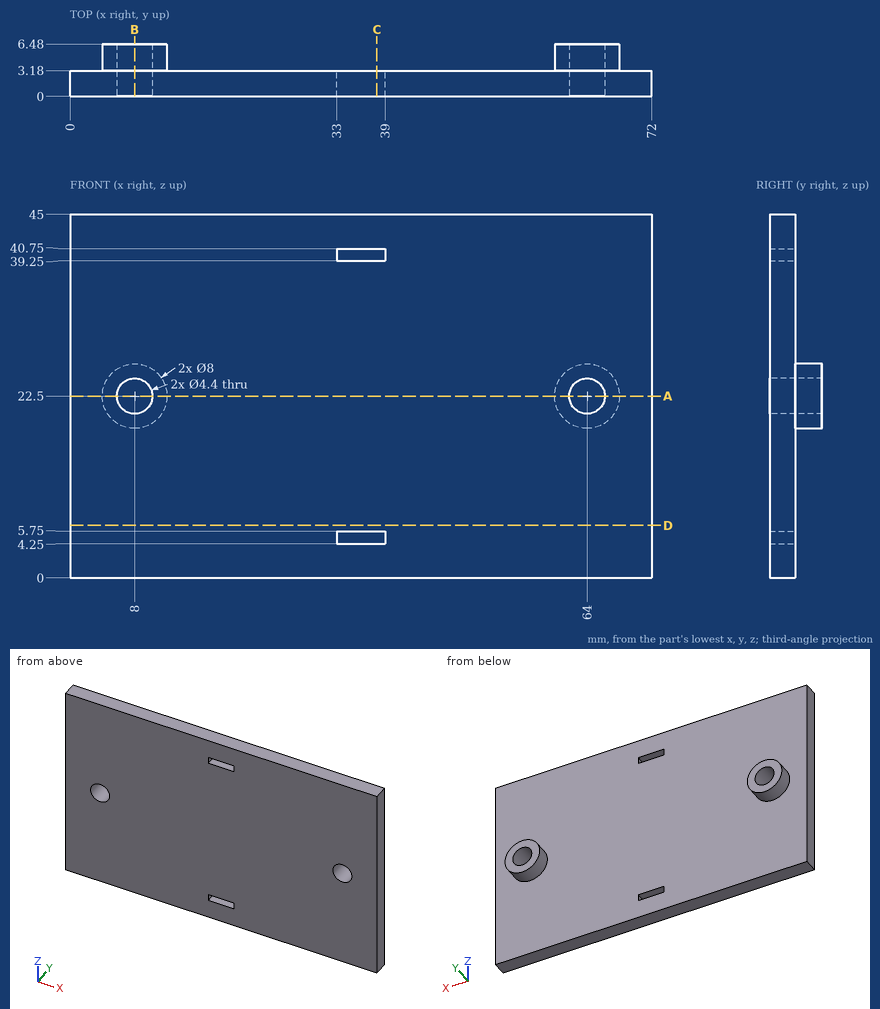
Verification items for this drawing (mm, ordinates from the low corner). Coordinates: 2 decimals unless noted, no trailing zeros. Write each loop counter-clockwise with the first axis right and the second up, starting at its lowest first coordinate (ties: lowest second). Pieces come first, ordered by that corner, then holes. Notation, with made-up numbers: (48, 4.25) -> (53, 4.25) arc R33 ccw to (53, 39.25) -> close; hole circle Ø2 at (-19, 41.5). An arc over 180 degrees is marked (long way). One line per item, written item: value. Start each with the question number.
Q1. Go/stop test with flat-tipped pins: P1, Ø13.5, axis at x = 20.5, z = 31, coming from the +Y side; P2, Ø4, axis at x = 51.5, z = 34, coming from the -Y side. Record where each tip stops, or that it passes through.
Q2. Cross-section at D-D on z = 6.5. Enter the section's corners in (x, y).
Q3. Cross-section at C-C on x = 38. Enter the section's corners in (y, z), and give its area (3 significant figures).
Q4. Thickness scan on L1, parallel to X at y = 2.75, z = 22.5; L2, parallel to X at y = 3.5, z = 22.5; L3, parallel to Z at x = 8, y = 2.25. Record the ranges inside material, lowest first. Write a range as from..to.
Q5. Cross-section at B-B on x = 8. Enter the section's corners in (y, z).
Q6. Cross-section at A-A on z = 22.5. Enter the section's corners in (x, y).
Checked values:
1. P1: stops at y = 3.18
1. P2: stops at y = 0
2. outline: (0, 0) -> (72, 0) -> (72, 3.18) -> (0, 3.18) -> close
3. outline: (0, 0) -> (3.18, 0) -> (3.18, 4.25) -> (0, 4.25) -> close; (0, 5.75) -> (3.18, 5.75) -> (3.18, 39.25) -> (0, 39.25) -> close; (0, 40.75) -> (3.18, 40.75) -> (3.18, 45) -> (0, 45) -> close
3. area: 134 mm²
4. L1: x = 0..5.8, 10.2..61.8, 66.2..72
4. L2: x = 4..5.8, 10.2..12, 60..61.8, 66.2..68
4. L3: z = 0..20.3, 24.7..45
5. outline: (0, 0) -> (3.18, 0) -> (3.18, 18.5) -> (6.48, 18.5) -> (6.48, 20.3) -> (0, 20.3) -> close; (0, 24.7) -> (6.48, 24.7) -> (6.48, 26.5) -> (3.18, 26.5) -> (3.18, 45) -> (0, 45) -> close
6. outline: (0, 0) -> (5.8, 0) -> (5.8, 6.48) -> (4, 6.48) -> (4, 3.18) -> (0, 3.18) -> close; (10.2, 0) -> (61.8, 0) -> (61.8, 6.48) -> (60, 6.48) -> (60, 3.18) -> (12, 3.18) -> (12, 6.48) -> (10.2, 6.48) -> close; (66.2, 0) -> (72, 0) -> (72, 3.18) -> (68, 3.18) -> (68, 6.48) -> (66.2, 6.48) -> close
